```python
from build123d import *

# Parameters (mm, degrees)
ESQUISSE1_W        = 43.6
ESQUISSE1_H        = 43.3
ESQUISSE1_R        = 1.5
BOSS_EXTRU_1_DEPTH = 2


with BuildPart() as part:
    # Esquisse1 → Boss.-Extru.1 (new body)
    with BuildSketch(Plane(origin=(0, 0, 0), x_dir=(1, 0, 0), z_dir=(0, 1, 0))):
        with Locations((21.8, 21.65)):
            Rectangle(ESQUISSE1_W, ESQUISSE1_H)
        with Locations(Location((3.3, 40, 0), (0, 0, 270))):
            Circle(ESQUISSE1_R, mode=Mode.SUBTRACT)
        with Locations(Location((40.3, 40, 0), (0, 0, 90))):
            Circle(ESQUISSE1_R, mode=Mode.SUBTRACT)
        with Locations(Location((40.3, 3.3, 0), (0, 0, 270))):
            Circle(ESQUISSE1_R, mode=Mode.SUBTRACT)
        with Locations(Location((3.3, 3.3, 0), (0, 0, 90))):
            Circle(ESQUISSE1_R, mode=Mode.SUBTRACT)
    extrude(amount=BOSS_EXTRU_1_DEPTH)


solid = part.part
```
Source: CAD feature listing. Evaluate the final solid. Frame: model axes, mm. Give positions to 0.01 mm unless a question says otherwise; leave off trailing zeros. Loops run counter-clockwise (first coordinate to the right, second up) from the corner with the lowest first, then second, coordinate; pieces in that order, holes last. Notation, with made-up numbers: (0.25, 5) - (4.25, 5) arc R21 ccw to (4.25, 9) - close; hole circle Ø5 at (-24.5, -11.75). An arc over 180 degrees is marked (long way). Use CSV: the item, a comma, the result in double quotes.
1) Pin query (flat end, axial travel): P1, Ø1.8, axis at x = 40.3, z = -3.3, coming from the +Y side (1 decimal); P2, Ø5, axis at x = 3.3, z = -3.3, coming from the -Y side. Return the tip coordinate at first contact, or that it passes through.
Worked out:
P1,"passes through"
P2,"stops at y = 0"
2) Line query: line 1 (X direction, y = 1, z = -3.3); line 2 (X direction, y = 1.9, z = -40.5). Output: solid intervals per line, ascending.
Worked out:
line 1,"x = 0 to 1.8, 4.8 to 38.8, 41.8 to 43.6"
line 2,"x = 0 to 1.89, 4.71 to 38.89, 41.71 to 43.6"
3) Mould query, pull axis Z, two halves, no side actions, for faces 1 (the flat face through (21, 1, -43.3)), 2 (the cylindrical face through (3.37, 0.99, -41.5)), 3 (the cylindrical face through (3.23, 0.99, -1.8)), 4 (the flat face through (0, 1, -21)). Classes: +Z half, -Z half, draft (parallel to the pull), parting line (faces both ways), or undercut.
Worked out:
face 1,"-Z half"
face 2,"undercut"
face 3,"undercut"
face 4,"draft"
4) Cut plane A-A (z = -3.3). Output: boundary loops of the cut face in (x, y).
Worked out:
outline,"(0, 0) - (1.8, 0) - (1.8, 2) - (0, 2) - close; (4.8, 0) - (38.8, 0) - (38.8, 2) - (4.8, 2) - close; (41.8, 0) - (43.6, 0) - (43.6, 2) - (41.8, 2) - close"
5) Cut plane B-B (x = 40.3). Output: boundary loops of the cut face in (y, z), and give its area (3 significant figures).
Worked out:
outline,"(0, -43.3) - (2, -43.3) - (2, -41.5) - (0, -41.5) - close; (0, -38.5) - (2, -38.5) - (2, -4.8) - (0, -4.8) - close; (0, -1.8) - (2, -1.8) - (2, 0) - (0, 0) - close"
area,"74.6 mm^2"
